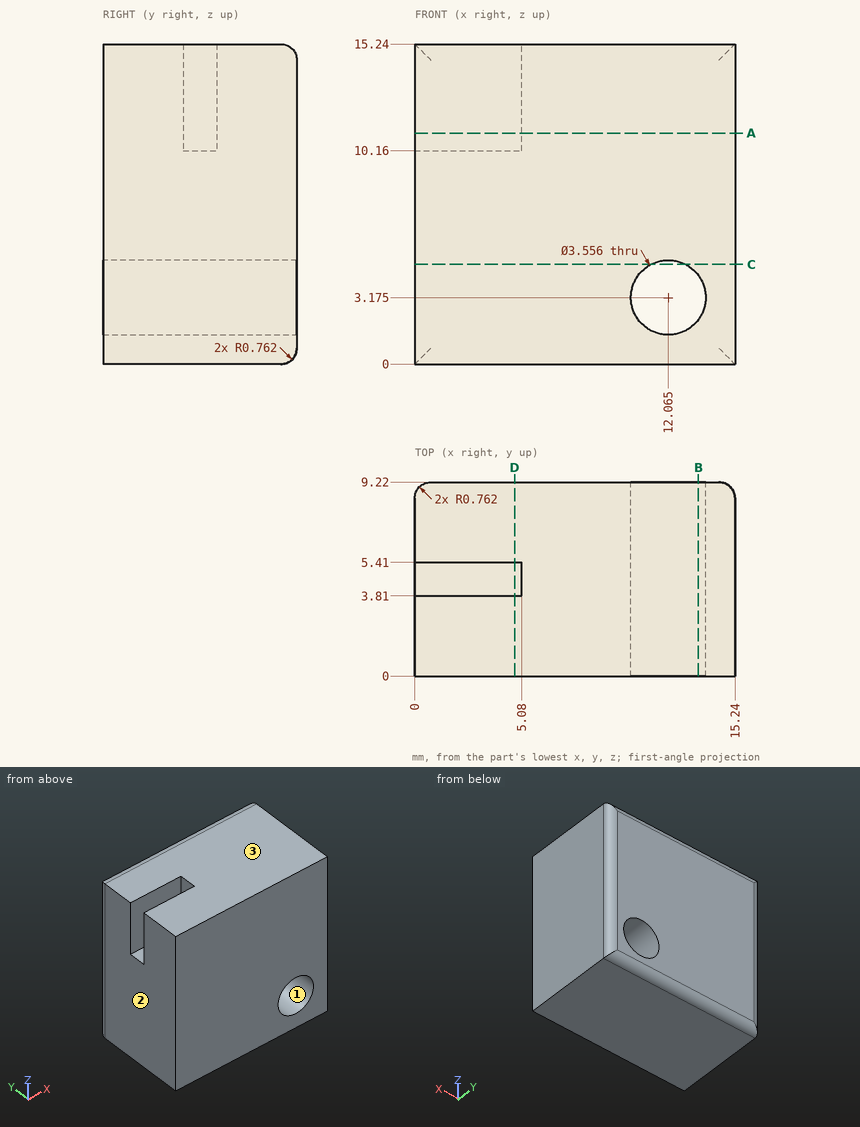
Print and shaded views of the part. All mm, measured from the part's lowest x, y and z. Give positions to 0.01 mm unless a question says otherwise; leave off trailing zeros. Loops run counter-clockwise (first coordinate to the right, second up) from the corner with the lowest first, then second, coordinate; pieces in that order, holes last. Notation, with made-up numbers: (-2, -8) -> (36, -8) arc R16 ccw to (36, 5) -> close; hole circle Ø8 at (51.5, 66.25). An arc over 180 degrees is marked (long way). Answer in a Markdown table with one row per item.
Item 1: Slice it at C-C on z = 4.75. Write the cut outline in (x, y), plus the area to 3 significant figures.
Findings below:
| item | result |
|---|---|
| outline | (0, 0) -> (11.24, 0) -> (11.24, 9.22) -> (0.76, 9.22) arc R0.76 ccw to (0, 8.46) -> close; (12.89, 0) -> (15.24, 0) -> (15.24, 8.46) arc R0.76 ccw to (14.48, 9.22) -> (12.89, 9.22) -> close |
| area | 125 mm² |
Item 2: Probe line 1 along Y through (x, z) = (2, 11.75); line 2 along X through (y, z) = (7.75, 3.25); line 3 along Z through (x, y) = (4.5, 5). List the from-to ranges inside material, lowest first. Write a range as [from, to].
Findings below:
| item | result |
|---|---|
| line 1 | y = [0, 3.81], [5.41, 9.22] |
| line 2 | x = [0, 10.29], [13.84, 15.24] |
| line 3 | z = [0, 10.16] |
Item 3: Flat gauge pins, fed straight in: P1, Ø1.3, axis at y = 4.5, z = 12, coming from the -X side; P2, Ø3, axis at x = 12.065, z = 3.175, coming from the +Y side. Where does each tip first touch, or does it go through?
Findings below:
| item | result |
|---|---|
| P1 | stops at x = 5.08 |
| P2 | passes through |
Item 4: Slice it at B-B on x = 13.5. Write the cut outline in (y, z) (1 decimal).
Findings below:
| item | result |
|---|---|
| outline | (0, 0) -> (8.5, 0) arc R0.8 ccw to (9.2, 0.8) -> (9.2, 2.1) -> (0, 2.1) -> close; (0, 4.2) -> (9.2, 4.2) -> (9.2, 14.5) arc R0.8 ccw to (8.5, 15.2) -> (0, 15.2) -> close |
Item 5: Mould opens along Z. For the marked faces 1, 2 and 3 say: pulls with the +Z half, pulls with the -Z half, needs draft (parallel to the pull), parting line crosses it, or undercut.
Findings below:
| item | result |
|---|---|
| face 1 | undercut |
| face 2 | needs draft |
| face 3 | pulls with the +Z half |
Item 6: Slice it at D-D on x = 4.75. Write the cut outline in (y, z), plus the area to 3 significant figures.
Findings below:
| item | result |
|---|---|
| outline | (0, 0) -> (8.46, 0) arc R0.76 ccw to (9.22, 0.76) -> (9.22, 14.48) arc R0.76 ccw to (8.46, 15.24) -> (5.41, 15.24) -> (5.41, 10.16) -> (3.81, 10.16) -> (3.81, 15.24) -> (0, 15.24) -> close |
| area | 132 mm² |
Item 7: Slice it at A-A on z = 11. Write the cut outline in (x, y), plus the area to 3 significant figures.
Findings below:
| item | result |
|---|---|
| outline | (0, 0) -> (15.24, 0) -> (15.24, 8.46) arc R0.76 ccw to (14.48, 9.22) -> (0.76, 9.22) arc R0.76 ccw to (0, 8.46) -> (0, 5.41) -> (5.08, 5.41) -> (5.08, 3.81) -> (0, 3.81) -> close |
| area | 132 mm² |
